Autodesk Inventor part; units mm, degrees
ref_plane "YZ Plane" through (0, 0, 0) normal (1, 0, 0) x (0, 1, 0)
ref_plane "XZ Plane" through (0, 0, 0) normal (0, 1, 0) x (-1, 0, 0)
ref_plane "XY Plane" through (0, 0, 0) normal (0, 0, 1) x (1, 0, 0)
sketch "Sketch1" plane through (0, 0, 0) normal (0, 1, 0) x (-1, 0, 0)
  line L0 (0, 0) -> (-176, 0)
  line L1 (-176, 0) -> (-176, -146)
  line L2 (-176, -146) -> (0, -146)
  line L3 (0, -146) -> (0, 0)
  line L4 (0, 0) -> (-176, 0)
  line L5 (-176, 0) -> (-176, -20)
  line L6 (-176, -20) -> (0, -20)
  line L7 (0, -20) -> (0, 0)
  line L8 (0, -146) -> (-20, -146)
  line L9 (-20, -146) -> (-20, 0)
  line L10 (-20, 0) -> (0, 0)
  line L11 (0, 0) -> (0, -146)
  line L12 (-20, -146) -> (-176, -146)
  line L13 (-176, -146) -> (-176, -143)
  line L14 (-176, -143) -> (-20, -143)
  line L15 (-20, -143) -> (-20, -146)
  line L16 (-20, -146) -> (-23, -146)
  line L17 (-23, -146) -> (-23, -20)
  line L18 (-23, -20) -> (-20, -20)
  line L19 (-20, -20) -> (-20, -146)
  line L20 (-20, -20) -> (-176, -20)
  line L21 (-176, -20) -> (-176, -23)
  line L22 (-176, -23) -> (-20, -23)
  line L23 (-20, -23) -> (-20, -20)
  line L24 (-176, -20) -> (-173, -20)
  line L25 (-173, -20) -> (-173, -146)
  line L26 (-173, -146) -> (-176, -146)
  line L27 (-176, -146) -> (-176, -20)
  line L28 (-20, -146) -> (-176, -146)
  line L29 (-176, -146) -> (-176, -143.2)
  line L30 (-176, -143.2) -> (-20, -143.2)
  line L31 (-20, -143.2) -> (-20, -146)
  line L32 (-176, -146) -> (-173.2, -146)
  line L33 (-173.2, -146) -> (-173.2, -20)
  line L34 (-173.2, -20) -> (-176, -20)
  line L35 (-176, -20) -> (-176, -146)
  line L36 (-176, -20) -> (-20, -20)
  line L37 (-20, -20) -> (-20, -22.8)
  line L38 (-20, -22.8) -> (-176, -22.8)
  line L39 (-176, -22.8) -> (-176, -20)
  line L40 (-20, -20) -> (-22.8, -20)
  line L41 (-22.8, -20) -> (-22.8, -146)
  line L42 (-22.8, -146) -> (-20, -146)
  line L43 (-20, -146) -> (-20, -20)
  line L44 (-23, -143) -> (-29, -143)
  line L45 (-29, -143) -> (-29, -137)
  line L46 (-29, -137) -> (-23, -137)
  line L47 (-23, -137) -> (-23, -143)
  line L48 (-173, -143) -> (-167, -143)
  line L49 (-167, -143) -> (-167, -137)
  line L50 (-167, -137) -> (-173, -137)
  line L51 (-173, -137) -> (-173, -143)
  line L52 (-173, -23) -> (-167, -23)
  line L53 (-167, -23) -> (-167, -29)
  line L54 (-167, -29) -> (-173, -29)
  line L55 (-173, -29) -> (-173, -23)
  line L56 (-23, -23) -> (-29, -23)
  line L57 (-29, -23) -> (-29, -29)
  line L58 (-29, -29) -> (-23, -29)
  line L59 (-23, -29) -> (-23, -23)
  line L60 (-23, -143) -> (-173, -143)
  line L61 (-173, -143) -> (-173, -23)
  line L62 (-173, -23) -> (-23, -23)
  line L63 (-23, -23) -> (-23, -143)
  circle A0 centre (-29, -137) radius 5
  circle A1 centre (-167, -137) radius 5
  circle A2 centre (-167, -29) radius 5
  circle A3 centre (-29, -29) radius 5
  line L64 (-22.8, -143.2) -> (-27.8, -143.2)
  line L65 (-27.8, -143.2) -> (-27.8, -138.2)
  line L66 (-27.8, -138.2) -> (-22.8, -138.2)
  line L67 (-22.8, -138.2) -> (-22.8, -143.2)
  line L68 (-173.2, -143.2) -> (-168.2, -143.2)
  line L69 (-168.2, -143.2) -> (-168.2, -138.2)
  line L70 (-168.2, -138.2) -> (-173.2, -138.2)
  line L71 (-173.2, -138.2) -> (-173.2, -143.2)
  line L72 (-173.2, -22.8) -> (-168.2, -22.8)
  line L73 (-168.2, -22.8) -> (-168.2, -27.8)
  line L74 (-168.2, -27.8) -> (-173.2, -27.8)
  line L75 (-173.2, -27.8) -> (-173.2, -22.8)
  line L76 (-22.8, -22.8) -> (-27.8, -22.8)
  line L77 (-27.8, -22.8) -> (-27.8, -27.8)
  line L78 (-27.8, -27.8) -> (-22.8, -27.8)
  line L79 (-22.8, -27.8) -> (-22.8, -22.8)
  circle A4 centre (-27.8, -138.2) radius 5
  circle A5 centre (-168.2, -138.2) radius 5
  circle A6 centre (-168.2, -27.8) radius 5
  circle A7 centre (-27.8, -27.8) radius 5
  dimension "d4" = 176
  dimension "d5" = 146
  dimension "d6" = 20
  dimension "d7" = 20
  dimension "d8" = 3
  dimension "d9" = 3
  dimension "d10" = 3
  dimension "d11" = 3
  dimension "d12" = 2.8
  dimension "d13" = 2.8
  dimension "d14" = 2.8
  dimension "d15" = 2.8
  dimension "d16" = 6
  dimension "d17" = 6
  dimension "d18" = 6
  dimension "d19" = 6
  dimension "d20" = 6
  dimension "d21" = 6
  dimension "d22" = 6
  dimension "d23" = 6
  dimension "d24" = 10
  dimension "d25" = 10
  dimension "d26" = 10
  dimension "d27" = 10
  dimension "d28" = 5
  dimension "d29" = 5
  dimension "d30" = 5
  dimension "d31" = 5
  dimension "d32" = 5
  dimension "d33" = 5
  dimension "d34" = 5
  dimension "d35" = 5
extrude "Extrusion1" add sketch "Sketch1" against normal blind 3
extrude "Extrusion2" add sketch "Sketch1" along normal blind 5 contours L77 L78 A3 L58 L57 | A3 L78 L77 | A7 A3 | A3 L57 L58 A7 | L74 L73 A2 L53 L54 | A2 L73 L74 | A6 A2 | A2 L54 L53 A6 | L66 L65 A0 L45 L46 | A0 L65 L66 | A4 A0 | A0 L46 L45 A4 | L70 L69 A1 | A1 L50 L49 L69 L70 | A5 A1 L49 L50 | A1 A5
extrude "Extrusion4" add sketch "Sketch1" along normal blind 6.5 contours L9 L38 L41 L6 | L6 L33 L38 L1 | L41 L38 L17 L6 | L9 L22 L41 L38 | L2 L41 L30 L9 | L38 L33 L22 L1 | L6 L25 L38 L33 | L17 L38 L25 L6 | L9 L14 L41 L22 | L2 L17 L30 L41 | L30 L41 L14 L9 | L22 L33 L14 L1 | L2 L25 L30 L17 | L14 L33 L30 L1 | L2 L33 L30 L25 | L30 L33 L2 L1
fillet "Fillet1" radius 5 4 edges at (22.8, 3.25, -143.2) (22.8, 3.25, -22.8) (173.2, 3.25, -22.8) (173.2, 3.25, -143.2)
sketch "Sketch2" plane through (29, 5, -137) normal (0, 1, 0) x (1, 0, 0)
  circle A0 centre (0, 0) radius 1.95
  circle A1 centre (138, 0) radius 5
  circle A2 centre (138, 0) radius 1.95
  circle A3 centre (138, -108) radius 5
  circle A4 centre (138, -108) radius 1.95
  circle A5 centre (0, -108) radius 5
  circle A6 centre (0, -108) radius 1.95
  point P0 (-29, -137)
  dimension "d45" = 3.9
  dimension "d46" = 3.9
  dimension "d47" = 3.9
  dimension "d48" = 3.9
extrude "Extrusion5" add sketch "Sketch2" along normal blind 8 contours A0 | A2 | A4 | A6
fillet "Fillet2" radius 5 4 edges at (176, 3.25, -20) (20, 3.25, -20) (176, 1.75, -146) (20, 3.25, -146)
fillet "Fillet3" radius 10 3 edges at (176, -1.5, 0) (0, -1.5, 0) (0, -1.5, -146)
sketch "Sketch3" plane through (0, 0, 0) normal (0, 1, 0) x (1, 0, 0)
  line L0 (25, 146) -> (10, 146)
  line L1 (0, 0) -> (20, 0)
  line L2 (20, 0) -> (20, 146)
  line L3 (20, 146) -> (0, 146)
  line L4 (0, 146) -> (0, 0)
  line L5 (176, 10) -> (176, 25)
  line L6 (0, 0) -> (176, 0)
  line L7 (176, 0) -> (176, 20)
  line L8 (176, 20) -> (0, 20)
  line L9 (0, 20) -> (0, 0)
  line L10 (20, 20) -> (0, 0)
  line L11 (20, 0) -> (0, 20)
  line L12 (176, 0) -> (156, 0)
  line L13 (156, 0) -> (156, 20)
  line L14 (156, 20) -> (176, 20)
  line L15 (176, 20) -> (176, 0)
  line L16 (0, 146) -> (20, 146)
  line L17 (20, 146) -> (20, 126)
  line L18 (20, 126) -> (0, 126)
  line L19 (0, 126) -> (0, 146)
  line L20 (20, 126) -> (0, 146)
  line L21 (20, 146) -> (0, 126)
  line L22 (176, 0) -> (156, 20)
  line L23 (156, 0) -> (176, 20)
  line L24 (166, 10) -> (10, 10)
  line L25 (10, 136) -> (10, 10)
  circle A0 centre (10, 136) radius 2.15
  circle A1 centre (10, 10) radius 2.15
  circle A2 centre (166, 10) radius 2.15
  dimension "d53" = 20
  dimension "d54" = 20
  dimension "d55" = 20
  dimension "d56" = 20
  dimension "d57" = 4.3
  dimension "d58" = 4.3
  dimension "d59" = 4.3
extrude "Extrusion6" cut sketch "Sketch3" against normal blind 8 contours A0 L20 L21 | L21 L20 A0 | A0 L25 L20 | L21 A0 L20 | L25 A0 L21 | A1 L24 L10 | L10 L25 A1 | A1 L11 L24 | A2 L23 L22 | L22 L24 A2 | L25 L11 A1 | L11 A1 L10 | L10 A1 L11 | L24 L23 A2 | A2 L22 L23 | L22 A2 L23
sketch "Sketch4" plane through (0, 6.5, 0) normal (0, 1, 0) x (1, 0, 0)
  arc A0 (20, 25) -> (25, 20) centre (25, 25) ccw
  line L0 (25, 20) -> (20, 20)
  line L1 (20, 20) -> (20, 25)
  line L2 (20, 25) -> (25, 25)
  line L3 (25, 25) -> (25, 20)
  line L4 (22.8, 27.8) -> (22.8, 138.2)
  line L5 (20, 20) -> (22.8, 20)
  line L6 (22.8, 20) -> (22.8, 34.25)
  line L7 (22.8, 34.25) -> (20, 34.25)
  line L8 (20, 34.25) -> (20, 20)
  line L9 (20, 34.25) -> (22.8, 34.25)
  line L10 (22.8, 34.25) -> (22.8, 46.25)
  line L11 (22.8, 46.25) -> (20, 46.25)
  line L12 (20, 46.25) -> (20, 34.25)
  point P0 (0, 0)
  dimension "d62" = 14.25
  dimension "d63" = 12
extrude "Extrusion7" cut sketch "Sketch4" against normal blind 2 contours L12 L11 L4 L7
properties part number "BottomCase"
CAD build for the part. Positions are in the model's coordinates, mm. A direction names the side the tool comes from. Give positions to 0.01 mm unless a question says otherwise; leave off trailing zeros. Order: outer loops, then holes, each group sorted by start corner. A loop starts at its lowest first (then second) coordinate and runs counter-clockwise, first axis right, second up. Notation, with made-up numbers: M -10.5,48 L -5.5,48 A17 cw -5.5,75 Z; hole C 60,3 d3. An arc over 180 degrees is marked long. Put each result on its own line as item: value. Start each with the question number.
(1) Mould opens along X. For faces 5 (the cylindrical face through (174, 2, -145)), 6 (the cylindrical face through (171.7, 3.3, -24.23)), 7 (the flat face through (29, 13, -137)) say: +X half, -X half, draft (parallel to the pull), parting line (faces both ways), or undercut.
(2) Saw through at B-B, the plane z = -113. Write the cut outline in (x, y), then the cut area to 3 significant figures.
(3) Saw through at C-C, the plane y = 9.5. Write the cut outline in (x, z).
(4) Saw through at A-A, the plane x = 40. Write the cut outline in (y, z).
(5) Flat gauge pins, fed straight in: pin 1 Ø7 at (x, y) = (102, 4.5) entering from +Z; pin 2 Ø12 at (x, z) = (65.5, -38.5) entering from +Y; pin 3 Ø2 at (y, z) = (3.5, -73) entering from -X. Where does each tip first touch, or does it go through?
(6) Which spindle directions (+Z, -Z, +X, -X, +Y, -Y) get a long thin tool onto all of the face, cutting with end or side? Do faces 1 (the flat face through (20, 3, -84)), 2 (the cylindrical face through (171.77, 3.3, -141.7)), 3 (the cylindrical face through (22, 3, -145)), 4 (the cylindrical face through (174, 3, -21)). Say none if no direction does.
(7) Drill centre lines: line 1 along X through (y, z) = (-1.3, -10); line 2 along Z through (x, y) = (84, 2.5); line 3 along Z through (x, y) = (166, -1.2). Where is each one in solid material? Low to high.
Check result:
1. face 5: +X half
1. face 6: undercut
1. face 7: draft
2. outline: M 0,-3 L 176,-3 L 176,6.5 L 173.2,6.5 L 173.2,0 L 22.8,0 L 22.8,6.5 L 20,6.5 L 20,0 L 0,0 Z
2. area: 564 mm2
3. outline: C 29,-137 d3.9; C 29,-29 d3.9; C 167,-137 d3.9; C 167,-29 d3.9
4. outline: M -3,-146 L 6.5,-146 L 6.5,-143.2 L 0,-143.2 L 0,-22.8 L 6.5,-22.8 L 6.5,-20 L 0,-20 L 0,0 L -3,0 Z
5. pin 1: stops at z = -20
5. pin 2: stops at y = 0
5. pin 3: stops at x = 20
6. face 1: +Z, -Z, -X, +Y
6. face 2: +Y
6. face 3: -Z, -X, +Y
6. face 4: +Z, +X, +Y
7. line 1: x = 0 to 7.85, 12.15 to 163.85, 168.15 to 176
7. line 2: z = -146 to -143.2, -22.8 to -20
7. line 3: z = -146 to -12.15, -7.85 to 0
